CAD build for the part. Positions are in the model's coordinates, mm. A direction names the side the tool comes from. Round coordinates to 2 decimals unless told otherwise and drop trailing zeros. Write each loop counter-clockwise with the first axis right and the second up, starting at its lowest first coordinate (ties: lowest second). Pieces come first, ordered by that corner, then holes. Notation, with made-up numbers: (77, 41.25) - (84, 41.25) arc R26 ccw to (84, 56.25) - close; hole circle Ø7 at (42, -36.75). An arc over 180 degrees is marked (long way). Answer in a Markdown table with one row per item.
```python
from build123d import *

# Parameters (mm, degrees)
SKETCH_W           = 100
SKETCH_H           = 50
PAD_DEPTH          = 3
SKETCH001_W        = 5
SKETCH001_H        = 5
PAD001_DEPTH       = 50
POLARPATTERN_COUNT = 2


with BuildPart() as part:
    # Sketch → Pad (new body)
    with BuildSketch(Plane.XY):
        Rectangle(SKETCH_W, SKETCH_H)
    extrude(amount=PAD_DEPTH)

    # Sketch001 (on Face5 of Pad) → Pad001 (join)
    with BuildSketch(Plane(origin=(0, 0, 0), x_dir=(1, 0, 0), z_dir=(0, 0, -1))):
        with Locations((44.5, 19.5)):
            Rectangle(SKETCH001_W, SKETCH001_H)
    pad001 = extrude(amount=PAD001_DEPTH)

    # Mirrored: Pad001 across Sketch001 V_Axis
    add(pad001.mirror(Plane(origin=(0, 0, 0), x_dir=(0, 0, -1), z_dir=(1, 0, 0))))

    # PolarPattern: Pad001 ×2 about axis
    polarpattern_axis = Axis((0, 0, 0), (0, 0, -1))
    for i in range(1, POLARPATTERN_COUNT):
        add(pad001.rotate(polarpattern_axis, i * 360 / POLARPATTERN_COUNT))

    # Mirrored001: Pad001 across Sketch001 H_Axis
    add(pad001.mirror(Plane(origin=(0, 0, 0), x_dir=(0, 0, -1), z_dir=(0, -1, 0))))


solid = part.part
```
Q1. Saw through at B-B on y = -20. List the corners of the cut face in (x, z), then the cut area to 3 significant figures.
Computed:
| item | result |
|---|---|
| outline | (-50, 0) - (-47, 0) - (-47, -50) - (-42, -50) - (-42, 0) - (42, 0) - (42, -50) - (47, -50) - (47, 0) - (50, 0) - (50, 3) - (-50, 3) - close |
| area | 800 mm2 |
Q2. Saw through at D-D on y = 10. List the corners of the cut face in (x, z).
Computed:
| item | result |
|---|---|
| outline | (-50, 0) - (50, 0) - (50, 3) - (-50, 3) - close |
Q3. 3-axis set-ups, long thin cutter, end or side, ignore diameter. For faces 1 (the flat face through (44, -17, -25)), 2 (the flat face through (-44, 22, -25)), 3 (the flat face through (47, -19, -25)): which of +Z, -Z, +X, -X, +Y, -Y reach the whole face in a straight line?
Computed:
| item | result |
|---|---|
| face 1 | -Z, +X, -X |
| face 2 | -Z, +X, -X, +Y |
| face 3 | -Z, +X, +Y, -Y |
Q4. Saw through at C-C on x = 28.5. List the corners of the cut face in (y, z), then the cut area to 3 significant figures.
Computed:
| item | result |
|---|---|
| outline | (-25, 0) - (25, 0) - (25, 3) - (-25, 3) - close |
| area | 150 mm2 |
Q5. Saw through at A-A on z = -40. List the corners of the cut face in (x, y), then the cut area to 3 significant figures.
Computed:
| item | result |
|---|---|
| outline | (-47, -22) - (-42, -22) - (-42, -17) - (-47, -17) - close; (-47, 17) - (-42, 17) - (-42, 22) - (-47, 22) - close; (42, -22) - (47, -22) - (47, -17) - (42, -17) - close; (42, 17) - (47, 17) - (47, 22) - (42, 22) - close |
| area | 100 mm2 |
Q6. Drill centre lines: line 1 (X direction, y = -20, z = -18); line 2 (Y direction, x = 45, z = -29.5); line 3 (Z direction, x = 16.5, y = 18). Where is each one in solid material? Low to high.
Computed:
| item | result |
|---|---|
| line 1 | x = -47 to -42, 42 to 47 |
| line 2 | y = -22 to -17, 17 to 22 |
| line 3 | z = 0 to 3 |
Q7. Flat gauge pins, fed straight in: pin 1 (4 mm diameter, centred on y = -20, z = -26.5, fed in from -X); pin 2 (5.5 mm diameter, centred on x = 45, z = -27.5, fed in from +Y); pin 3 (2.5 mm diameter, centred on x = 44.5, z = -28, fed in from -Y). Where does each tip first touch, or does it go through?
Computed:
| item | result |
|---|---|
| pin 1 | stops at x = -47 |
| pin 2 | stops at y = 22 |
| pin 3 | stops at y = -22 |
Q8. Pull direction Y, two halves, no side cores. Call faces 4 (the flat face through (-44, -22, -25)), 5 (the flat face through (44, 17, -25)), 6 (the flat face through (-44, 17, -25)), 7 (the flat face through (44, 20, -50)): released by +Y, released by -Y, zero draft, split by the parting line, or undercut.
Computed:
| item | result |
|---|---|
| face 4 | released by -Y |
| face 5 | undercut |
| face 6 | undercut |
| face 7 | zero draft |
